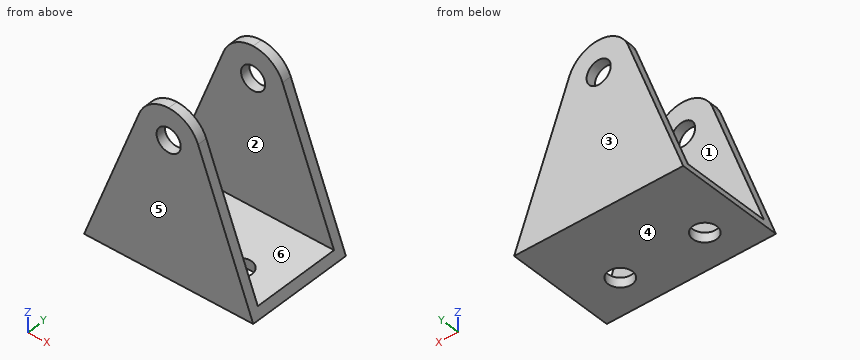
from build123d import *

# Parameters (mm, degrees)
SKETCH1_W               = 70
SKETCH1_H               = 45
SKETCH1_R               = 5
BOSS_EXTRUDE1_DEPTH     = 70
SKETCH2_R               = 5
CUT_EXTRUDE1_DEPTH      = 70
CUT_EXTRUDE2_DEPTH      = 181.24938524
CUT_EXTRUDE2_DEPTH_BACK = 181.24938524
SKETCH3_W               = 72.235560481
SKETCH3_H               = 37


with BuildPart() as part:
    # Sketch1 → Boss-Extrude1 (new body)
    with BuildSketch(Plane.XY.offset(32.9)):
        with Locations((0.858254713, 121.799876296)):
            Rectangle(SKETCH1_W, SKETCH1_H)
        with Locations((-17.5, 114.3)):
            Circle(SKETCH1_R, mode=Mode.SUBTRACT)
        with Locations((17.5, 114.3)):
            Circle(SKETCH1_R, mode=Mode.SUBTRACT)
    extrude(amount=BOSS_EXTRUDE1_DEPTH)

    # Sketch2 → Cut-Extrude1 (cut)
    with BuildSketch(Plane(origin=(0, 144.299876296, 0), x_dir=(1, 0, 0), z_dir=(0, 1, 0))):
        with BuildLine():
            Line((0.858254713, -101.89), (0.858254713, -102.9))
            Line((0.858254713, -102.9), (35.858254713, -102.9))
            Line((35.858254713, -102.9), (35.858254713, -32.9))
            Line((35.858254713, -32.9), (13.022608826, -93.475683049))
            ThreePointArc((13.022608826, -93.475683049), (8.253730369, -99.581442364), (0.858254713, -101.89))
        make_face()
        with BuildLine():
            Line((-34.141745287, -102.9), (0.858254713, -102.9))
            Line((0.858254713, -102.9), (0.858254713, -101.89))
            ThreePointArc((0.858254713, -101.89), (-6.537220943, -99.581442364), (-11.306099399, -93.475683049))
            Line((-11.306099399, -93.475683049), (-34.141745287, -32.9))
            Line((-34.141745287, -32.9), (-34.141745287, -102.9))
        make_face()
        with Locations(Location((0.858254713, -88.89, 0), (0, 0, 270))):
            Circle(SKETCH2_R)
    extrude(amount=-CUT_EXTRUDE1_DEPTH, mode=Mode.SUBTRACT)

    # Sketch3 → Cut-Extrude2 (cut, two sides: drawn at the far end of the back side and taken through both)
    with BuildSketch(Plane(origin=(0, 0, 0), x_dir=(0, 0, -1), z_dir=(1, 0, 0)).offset(-CUT_EXTRUDE2_DEPTH_BACK)):
        with Locations((-73.017780241, 121.799876296)):
            Rectangle(SKETCH3_W, SKETCH3_H)
    extrude(amount=CUT_EXTRUDE2_DEPTH + CUT_EXTRUDE2_DEPTH_BACK, mode=Mode.SUBTRACT)


solid = part.part
Could you check a few things on this model? Use its own coordinates, in mm. Face numbers are marked on the shaded views. A direction names the side the tool comes from. Give positions to 0.01 mm unless a question says otherwise; leave off trailing zeros. Order: outer loops, then holes, each group sorted by start corner. A loop starts at its lowest first (then second) coordinate and runs counter-clockwise, first axis right, second up. Notation, with made-up numbers: (75.5, -34) - (108.5, -34) arc R10 cw to (108.5, -25) - close; hole circle Ø6 at (41, 42.25). An arc over 180 degrees is marked (long way). One line per item, written item: value. Start each with the question number.
1. Imagine slicing it at D-D on z = 51. List the corners of the cut face in (x, y) for me, plus the area to 3 significant figures.
2. If I drill on probe 1 along Y at (x, z) = (-13, 87); probe 2 along Y at (x, z) = (-17.5, 34); probe 3 along Z at (x, y) = (8.5, 107), over which ranges is the centre line in solid material (lowest first)?
3. Imagine slicing it at C-C on z = 88.89. List the corners of the cut face in (x, y) for me.
4. Imagine slicing it at B-B on x = -17.5. List the corners of the cut face in (y, z) for me, plus the area to 3 significant figures.
5. Thinking about a two-plate mould opening in Y: for the marked faces 1, 2, 3 and 4, which applies, +Y half, -Y half, draft (parallel to the pull), parting line (faces both ways), or undercut?
6. For P1, Ø3, axis at y = 138.5, z = 80.5, coming from the -X side; P2, Ø13, axis at x = 17.5, y = 114.3, coming from the +Z side, each with a flat end and sliding along its axis, tell me the tip position at first contact or that it passes through.
7. Imagine slicing it at A-A on y = 114.3. List the corners of the cut face in (x, z) for me.
8. For the marked faces 5 and 6, which set-ups out of +Z, -Z, +X, -X, +Y, -Y let a thin tool reach every point of the face, with its end or its side?
Values:
1. outline: (-27.32, 99.3) - (29.03, 99.3) - (29.03, 103.3) - (-27.32, 103.3) - close; (-27.32, 140.3) - (29.03, 140.3) - (29.03, 144.3) - (-27.32, 144.3) - close
1. area: 451 mm²
2. probe 1: 99.3 to 103.3, 140.3 to 144.3
2. probe 2: 99.3 to 109.3, 119.3 to 144.3
2. probe 3: 32.9 to 36.9
3. outline: (-13.03, 99.3) - (-4.14, 99.3) - (-4.14, 103.3) - (-13.03, 103.3) - close; (-13.03, 140.3) - (-4.14, 140.3) - (-4.14, 144.3) - (-13.03, 144.3) - close; (5.86, 99.3) - (14.75, 99.3) - (14.75, 103.3) - (5.86, 103.3) - close; (5.86, 140.3) - (14.75, 140.3) - (14.75, 144.3) - (5.86, 144.3) - close
4. outline: (99.3, 32.9) - (109.3, 32.9) - (109.3, 36.9) - (103.3, 36.9) - (103.3, 77.05) - (99.3, 77.05) - close; (119.3, 32.9) - (144.3, 32.9) - (144.3, 77.05) - (140.3, 77.05) - (140.3, 36.9) - (119.3, 36.9) - close
4. area: 461 mm²
5. face 1: undercut
5. face 2: undercut
5. face 3: +Y half
5. face 4: draft
6. P1: through
6. P2: z = 36.9
7. outline: (-34.14, 32.9) - (-22.5, 32.9) - (-22.5, 36.9) - (-32.63, 36.9) - close; (-12.5, 32.9) - (12.5, 32.9) - (12.5, 36.9) - (-12.5, 36.9) - close; (22.5, 32.9) - (35.86, 32.9) - (34.35, 36.9) - (22.5, 36.9) - close
8. face 5: +Z, -Z, +X, -X, -Y
8. face 6: +Z, +X, -X
